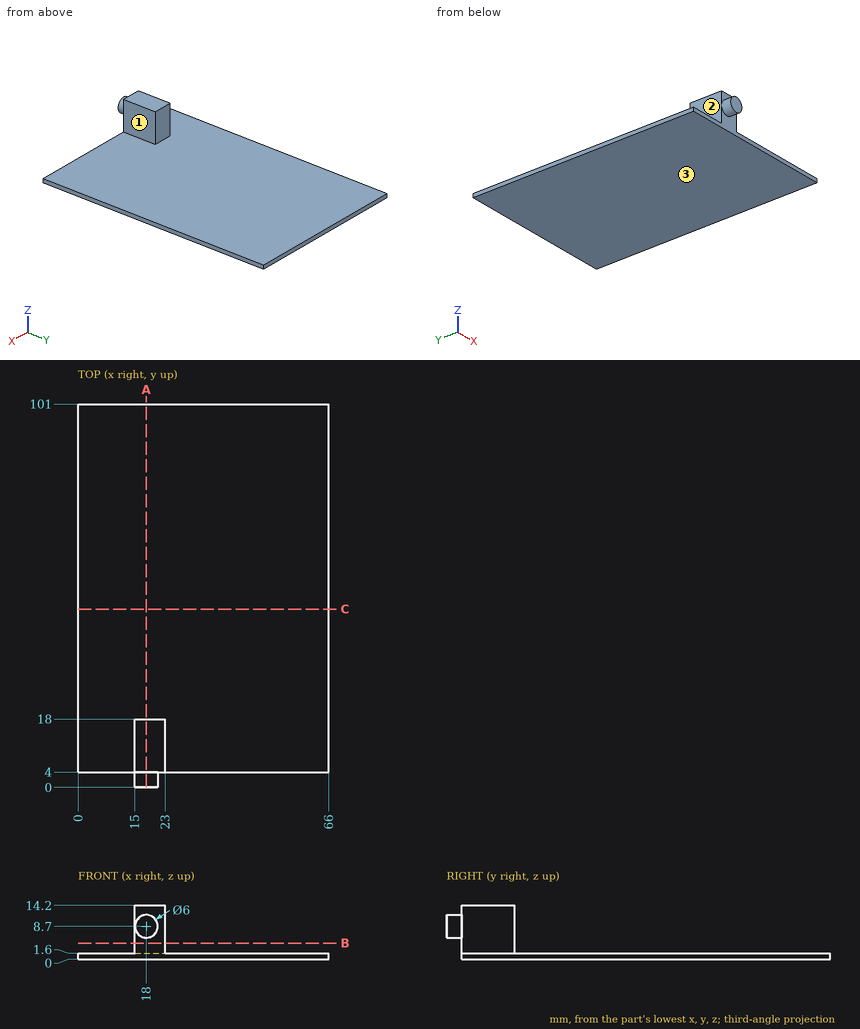
Geometry: see drawing. Coordinates: mm, zero at the bounding-box minimum. A direction names the side the tool comes from. Round coordinates to 2 decimals unless told otherwise and drop trailing zeros. Order: outer loops, then holes, each group sorted by start corner. A loop starts at its lowest first (then second) coordinate and runs counter-clockwise, first axis right, second up. Notation, with made-up numbers: (7, 38) -> (23, 38) arc R19 ccw to (23, 68) -> close; hole circle Ø8 at (17, 67). An arc over 180 degrees is marked (long way). Write each question's results on one line, items separated by ' | '.
Q1. Pin query (flat end, axial travel): pin 1 Ø6.5 at (y, z) = (9.5, 10.5) entering from -X; pin 2 Ø1 at (x, y) = (9, 88.5) entering from +Z. Return the tip coordinate at first contact, or that it passes through.
Response values:
pin 1: x = 15 | pin 2: z = 1.6
Q2. Section query A-A (x = 18). Output: boundary loops of the cut face in (y, z).
Response values:
outline: (0, 5.7) -> (4, 5.7) -> (4, 0) -> (101, 0) -> (101, 1.6) -> (18, 1.6) -> (18, 14.2) -> (4, 14.2) -> (4, 11.7) -> (0, 11.7) -> close
Q3. Access query for the marked faces 1, 2 and 3. Directions: +Z, -Z, +X, -X, +Y, -Y. A direction counts if a zero-diameter tool reaches every point of the face in a straight line with its end or side. Return the directions, or none.
Response values:
face 1: +Z, +X, +Y, -Y | face 2: +Z, -X, +Y, -Y | face 3: -Z, +X, -X, +Y, -Y
Q4. Ray query, line 1 along Z through (x, y) = (20.5, 86); line 2 along X through (y, z) = (10, 5.75); line 3 along Y through (x, z) = (22, 13.5). Return the intervals inside material, ascending.
Response values:
line 1: 0 to 1.6 | line 2: 15 to 23 | line 3: 4 to 18
Q5. Section query C-C (y = 47). Output: boundary loops of the cut face in (x, z), and give its area (3 significant figures).
Response values:
outline: (0, 0) -> (66, 0) -> (66, 1.6) -> (0, 1.6) -> close | area: 106 mm²
Q6. Section query B-B (z = 4.25). Output: boundary loops of the cut face in (x, y).
Response values:
outline: (15, 4) -> (23, 4) -> (23, 18) -> (15, 18) -> close
